```python
from build123d import *

# Parameters (mm, degrees)
SKETCH1_R                = 25
SKETCH1_R_2              = 18
BOSS_EXTRUDE1_DEPTH      = 80
SKETCH2_W                = 12
SKETCH2_H                = 40
BOSS_EXTRUDE2_DEPTH      = 13
BOSS_EXTRUDE3_REACH      = 99.596
BOSS_EXTRUDE3_END_RADIUS = 25
SKETCH4_W                = 26
SKETCH4_H                = 40
SKETCH5_R                = 10
CUT_EXTRUDE1_DEPTH       = 106.32331176
BOSS_EXTRUDE4_DEPTH      = 10
SKETCH6_3_R              = 20
BOSS_EXTRUDE5_DEPTH      = 20
BOSS_EXTRUDE6_REACH      = 119.256
BOSS_EXTRUDE6_END_RADIUS = 25
SKETCH7_W                = 20
SKETCH7_H                = 40
SKETCH8_R                = 12.5
CUT_EXTRUDE2_DEPTH       = 120.808180021
RIB2_START               = -5
RIB2_DEPTH               = 10
SKETCH10_W               = 67.322464705
SKETCH10_H               = 6
CUT_EXTRUDE3_DEPTH       = 114.815640401


with BuildPart() as part:
    # Sketch1 → Boss-Extrude1 (new body)
    with BuildSketch(Plane(origin=(0, 0, 0), x_dir=(1, 0, 0), z_dir=(0, 1, 0))):
        with Locations(Location((0, 0, 0), (0, 0, 270))):
            Circle(SKETCH1_R)
        with Locations(Location((0, 0, 0), (0, 0, 270))):
            Circle(SKETCH1_R_2, mode=Mode.SUBTRACT)
    extrude(amount=BOSS_EXTRUDE1_DEPTH)



with BuildPart() as body_2:
    # Sketch2 → Boss-Extrude2 (new, symmetric)
    with BuildSketch(Plane.XY):
        with BuildLine():
            Line((-37, 80), (-37, 40))
            ThreePointArc((-37, 40), (-57, 60), (-37, 80))
        make_face()
        with Locations((-31, 60)):
            Rectangle(SKETCH2_W, SKETCH2_H)
    extrude(amount=BOSS_EXTRUDE2_DEPTH, both=True)


with BuildPart() as part_1:
    add(part.part)

    add(body_2.part)  # Boss-Extrude3 merges body 2
    # Boss-Extrude3: up to this cylinder (the profile starts outside it)
    boss_extrude3_end = Plane(origin=(0, 60, 0), z_dir=(0, -1, 0)) * Cylinder(BOSS_EXTRUDE3_END_RADIUS, 250.192, mode=Mode.PRIVATE)
    # Sketch4 → Boss-Extrude3 (add, up to the surface)
    with BuildSketch(Plane(origin=(-25, 0, 0), x_dir=(0, 0, -1), z_dir=(1, 0, 0)), mode=Mode.PRIVATE) as boss_extrude3_sk1:
        with Locations((0, 60)):
            Rectangle(SKETCH4_W, SKETCH4_H)
    boss_extrude3_tool1 = extrude(boss_extrude3_sk1.sketch, amount=BOSS_EXTRUDE3_REACH, mode=Mode.PRIVATE) - boss_extrude3_end
    add(boss_extrude3_tool1.solids().sort_by_distance((-25, 60, 0))[0])
    add(boss_extrude3_tool1.solids().sort_by_distance((-25, 60, 0))[1])

    # Sketch5 → Cut-Extrude1 (cut, through all)
    with BuildSketch(Plane.XY.offset(13)):
        with Locations((-37, 60)):
            Circle(SKETCH5_R)
    extrude(amount=-CUT_EXTRUDE1_DEPTH, mode=Mode.SUBTRACT)



with BuildPart() as body_2_2:
    # Sketch6 → Boss-Extrude4 (new, symmetric)
    with BuildSketch(Plane.XY):
        with BuildLine():
            Line((25, 40), (25, 0))
            Line((25, 0), (57, 0))
            ThreePointArc((57, 0), (37, 20), (57, 40))
            Line((57, 40), (25, 40))
        make_face()
    extrude(amount=BOSS_EXTRUDE4_DEPTH, both=True)

    # Sketch6<3> → Boss-Extrude5 (add, symmetric)
    with BuildSketch(Plane.XY):
        with Locations((57, 20)):
            Circle(SKETCH6_3_R)
    extrude(amount=BOSS_EXTRUDE5_DEPTH, both=True)


with BuildPart() as part_2:
    add(part_1.part)

    add(body_2_2.part)  # Boss-Extrude6 merges body 2 2
    # Boss-Extrude6: up to this cylinder (the profile starts outside it)
    boss_extrude6_end = Plane(origin=(0, 20, 0), z_dir=(0, -1, 0)) * Cylinder(BOSS_EXTRUDE6_END_RADIUS, 289.512, mode=Mode.PRIVATE)
    # Sketch7 → Boss-Extrude6 (add, up to the surface)
    with BuildSketch(Plane.ZY.offset(-25), mode=Mode.PRIVATE) as boss_extrude6_sk1:
        with Locations((0, 20)):
            Rectangle(SKETCH7_W, SKETCH7_H)
    boss_extrude6_tool1 = extrude(boss_extrude6_sk1.sketch, amount=BOSS_EXTRUDE6_REACH, mode=Mode.PRIVATE) - boss_extrude6_end
    add(boss_extrude6_tool1.solids().sort_by_distance((25, 20, 0))[0])
    add(boss_extrude6_tool1.solids().sort_by_distance((25, 20, 0))[1])

    # Sketch8 → Cut-Extrude2 (cut, through all)
    with BuildSketch(Plane.XY.offset(20)):
        with Locations((57, 20)):
            Circle(SKETCH8_R)
    extrude(amount=-CUT_EXTRUDE2_DEPTH, mode=Mode.SUBTRACT)

    # Rib2: read off the stored shape, not the designer's step
    # Rib2 outline → Rib2 (add)
    with BuildSketch(Plane.XY.offset(RIB2_START)):
        Polygon((25, 80), (24.494897428, 80), (24.494897428, 40), (45, 40), align=None)
    extrude(amount=RIB2_DEPTH)

    # Sketch10 → Cut-Extrude3 (cut, through all)
    with BuildSketch(Plane(origin=(0, 80, 0), x_dir=(1, 0, 0), z_dir=(0, 1, 0))):
        with Locations((-36.448129058, 0)):
            Rectangle(SKETCH10_W, SKETCH10_H)
    extrude(amount=-CUT_EXTRUDE3_DEPTH, mode=Mode.SUBTRACT)


solid = part_2.part
```
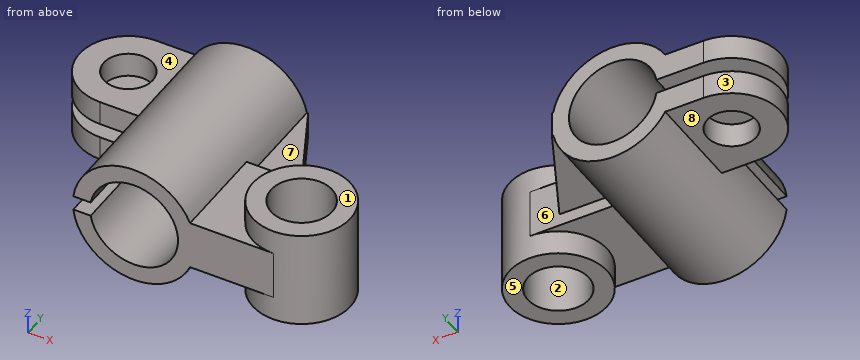
Input: part model. Units: mm. Frame: model coordinates. Face numbers are marked on the shaded views. A direction names the side the tool comes from. Coordinates: 2 decimals unless noted, no trailing zeros. Write each loop counter-clockwise with the first axis right and the second up, starting at its lowest first coordinate (ties: lowest second). Pieces come first, ordered by that corner, then holes.
1) Set-up query: the marked faces 4, 5, 6, 7 and 8. Return all of +Z, -Z, +X, -X, +Y, -Y with unobstructed straight access to the full face (end or side cutting, diameter ignored); none if empty.
2) Section D-D on z = 0. Output: boundary loops of the cut face in (x, y).
3) Mould query, pull axis X, two halves, no side actions, for the marked faces 1, 2 and 3. Classes: pulls with the +X half, pulls with the -X half, needs draft (parallel to the pull), parting line crosses it, or undercut.
4) Section A-A on x = 0. Output: boundary loops of the cut face in (y, z).
5) Pin query (flat end, axial travel): pin 1 Ø12 at (x, y) = (48, 13) entering from +Z; pin 2 Ø15 at (x, y) = (57, 20) entering from +Z; pin 3 Ø3 at (x, z) = (-30, 9) entering from -Y; pin 4 Ø5 at (x, y) = (17, 28) entering from +Z. Return the tip coordinate at first contact, or that it passes through.
6) Section C-C on y = 60. Output: boundary loops of the cut face in (x, z).
7) Section B-B on y = 20. Output: boundary loops of the cut face in (x, z).
8) Material intervals for line 1 along Z through (x, y) = (-42, 76); line 2 along Y through (x, z) = (57, 8); line 3 along Z through (x, y) = (0, 22), sorted ascending.
Check result:
1. face 4: +Z, -X, +Y, -Y
1. face 5: -Z, +X, +Y, -Y
1. face 6: +X, +Y
1. face 7: +Z, +X, +Y
1. face 8: -Z, -X, +Y, -Y
2. outline: (18, 0) - (57, 0) arc R20 ccw to (57, 40) - (45, 40) - (25, 80) - (18, 80) - close; hole circle Ø25 at (57, 20)
3. face 1: needs draft
3. face 2: undercut
3. face 3: pulls with the -X half
4. outline: (0, -25) - (80, -25) - (80, -18) - (0, -18) - close; (0, 18) - (80, 18) - (80, 25) - (0, 25) - close
5. pin 1: stops at z = 20
5. pin 2: passes through
5. pin 3: stops at y = 40
5. pin 4: stops at z = 20.37
6. outline: (-57, -13) - (-47, -13) - (-47, -3) - (-57, -3) - close; (-57, 3) - (-47, 3) - (-47, 13) - (-57, 13) - close; (-27, -13) - (-21.35, -13) arc R25 ccw to (24.49, -5) - (35, -5) - (35, 5) - (24.49, 5) arc R25 ccw to (-21.35, 13) - (-27, 13) - (-27, 3) - (-17.75, 3) arc R18 cw (long way) to (-17.75, -3) - (-27, -3) - close
7. outline: (-24.82, -3) arc R25 ccw to (22.91, -10) - (37, -10) - (37, -20) - (44.5, -20) - (44.5, 20) - (37, 20) - (37, 10) - (22.91, 10) arc R25 ccw to (-24.82, 3) - (-17.75, 3) arc R18 cw (long way) to (-17.75, -3) - close; (69.5, -20) - (77, -20) - (77, 20) - (69.5, 20) - close
8. line 1: z = -13 to -3, 3 to 13
8. line 2: y = 0 to 7.5, 32.5 to 40
8. line 3: z = -25 to -18, 18 to 25
